Check sheet for the modelled part. Datum: model origin and axes. Units: mm. A direction names the side the tool comes from. Round coordinates to 2 decimals unless told otherwise and drop trailing zeros. Loops run counter-clockwise (first coordinate to the right, second up) from the corner with the lowest first, then second, coordinate; pieces in that order, holes last. Notation, with made-up numbers: (-6.75, 53.25) - (36.25, 53.25) arc R29 cw to (36.25, 91.25) - close; hole circle Ø8 at (-6, 54.25). An arc over 180 degrees is marked (long way). Answer in a Markdown table with one row per item. Add a question column.
(1) Mould release check, pull along Z, two halves, no side actions. Record for faces 5 (the flat face through (-1, -30, 101.6)), 6 (the flat face through (7, 38, 88.9)), 7 (the flat face through (25.4, 0, 52)): +Z half, -Z half, draft (parallel to the pull), parting line (faces both ways), or undercut.
(2) Cross-section at A-A on y = 0. Enter the section's corners in (x, z), then the cut area to 3 significant figures.
(3) Thickness scan on line 1 along Z through (x, y) = (-37, -17); line 2 along Z through (x, y) = (-9.5, -57.5); line 3 along Z through (x, y) = (-49, -6.5). Record the ranges inside material, lowest first.
(4) Access from +Z, -Z, +X, -X, +Y, -Y to the whole of each face (thin tool, end or side, straight path). Record for faces 1 (the cylindrical face through (-44.833, -1.907, 6.261)), 2 (the flat face through (0, 25.4, 52)), 3 (the cylindrical face through (-11.012, -49.592, 92.657)), 4 (the flat face through (27.3, -27.3, 12.7)).
(5) Gauge pin test, flat ends, axial feed: pin 1 (7.5 mm diameter, centred on x = 0, y = 50.51, fed in from +Z); pin 2 (6 mm diameter, centred on x = 35, z = 41.5, fed in from +Y); pin 3 (6 mm diameter, centred on y = 0.5, z = 32.5, fed in from -X). Record the tip position at first contact, or that the pin passes through.
(6) Cross-section at B-B on x = -52.5. Enter the section's corners in (y, z).
(7) Cross-section at C-C on z = 79. Enter the section's corners in (x, y).
from build123d import *

# Parameters (mm, degrees)
F0_R      = 63.5
F1_DEPTH  = 12.7
F2_R      = 31.75
F3_DEPTH  = 76.2
F4_R      = 38.1
F5_DEPTH  = 76.2
F6_R      = 50.8
F7_DEPTH  = 12.7
F8_R      = 5.08
F9_R      = 6.35
F10_DEPTH = 50.8
F11_W     = 50.8
F11_H     = 50.8
F12_DEPTH = 120.142


with BuildPart() as f1:
    # F0 (on Top) → F1 (new body)
    with BuildSketch(Plane.XY):
        Circle(F0_R)
    extrude(amount=F1_DEPTH)

    # F2 (on face) → F3 (cut)
    with BuildSketch(Plane.XY.offset(12.7)):
        Circle(F2_R)
    extrude(amount=F3_DEPTH, mode=Mode.SUBTRACT)

    # F4 (on face) → F5 (join)
    with BuildSketch(Plane.XY.offset(12.7)):
        Circle(F4_R)
    extrude(amount=F5_DEPTH)

    # F6 (on face) → F7 (join)
    with BuildSketch(Plane.XY.offset(88.9)):
        Circle(F6_R)
    extrude(amount=F7_DEPTH)

    # F8
    f8_edges = [f1.edges().sort_by_distance(p)[0] for p in [
        (-50.8, 0, 101.6),
    ]]
    fillet(f8_edges, radius=F8_R)

    # F9 (on face) → F10 (cut)
    with BuildSketch(Plane(origin=(0, 0, 0), x_dir=(1, 0, 0), z_dir=(0, 0, -1))):
        with BuildLine():
            ThreePointArc((57.239421, 0), (50.889421, 6.35), (44.539421, 0))
            ThreePointArc((44.539421, 0), (50.889421, -6.35), (57.239421, 0))
        make_face()
        with BuildLine():
            ThreePointArc((6.35, -50.507508), (4.490128, -46.01738), (0, -44.157508))
            ThreePointArc((0, -44.157508), (-4.490128, -54.997636), (6.35, -50.507508))
        make_face()
        with Locations((-50.889418, 0)):
            Circle(F9_R)
        with BuildLine():
            ThreePointArc((6.35, 51.080368), (-4.490128, 55.570497), (0, 44.730368))
            ThreePointArc((0, 44.730368), (4.490128, 46.59024), (6.35, 51.080368))
        make_face()
    extrude(amount=-F10_DEPTH, mode=Mode.SUBTRACT)

    # F11 (on face) → F12 (cut)
    with BuildSketch(Plane.XY.offset(101.6)):
        Rectangle(F11_W, F11_H)
    extrude(amount=-F12_DEPTH, mode=Mode.SUBTRACT)


solid = f1.part
Answers:
| question | item | result |
|---|---|---|
| 1 | face 5 | +Z half |
| 1 | face 6 | undercut |
| 1 | face 7 | draft |
| 2 | outline | (-63.5, 0) - (-57.24, 0) - (-57.24, 12.7) - (-63.5, 12.7) - close; (-50.8, 88.9) - (-38.1, 88.9) - (-38.1, 12.7) - (-44.54, 12.7) - (-44.54, 0) - (-25.4, 0) - (-25.4, 101.6) - (-45.72, 101.6) arc R5.08 ccw to (-50.8, 96.52) - close; (25.4, 0) - (44.54, 0) - (44.54, 12.7) - (38.1, 12.7) - (38.1, 88.9) - (50.8, 88.9) - (50.8, 96.52) arc R5.08 ccw to (45.72, 101.6) - (25.4, 101.6) - close; (57.24, 0) - (63.5, 0) - (63.5, 12.7) - (57.24, 12.7) - close |
| 2 | area | 3,210 mm^2 |
| 3 | line 1 | z = 0 to 12.7, 88.9 to 101.6 |
| 3 | line 2 | z = 0 to 12.7 |
| 3 | line 3 | z = 0 to 12.7, 88.9 to 99.99 |
| 4 | face 1 | -Z |
| 4 | face 2 | +Z, -Z |
| 4 | face 3 | +Z |
| 4 | face 4 | none |
| 5 | pin 1 | stops at z = 101.49 |
| 5 | pin 2 | stops at y = 20.68 |
| 5 | pin 3 | stops at x = -38.1 |
| 6 | outline | (-35.72, 0) - (-6.14, 0) - (-6.14, 12.7) - (-35.72, 12.7) - close; (6.14, 0) - (35.72, 0) - (35.72, 12.7) - (6.14, 12.7) - close |
| 7 | outline | circle Ø76.2 at (0, 0); hole (-25.4, -25.4) - (25.4, -25.4) - (25.4, 25.4) - (-25.4, 25.4) - close |
